Design review of the part built by this model. Coordinates are the model's own, in mm. A direction names the side the tool comes from. Give positions to 0.01 mm unless a question says otherwise; leave off trailing zeros. Order: outer loops, then holes, each group sorted by start corner. A loop starts at its lowest first (then second) coordinate and runs counter-clockwise, first axis right, second up. Notation, with made-up numbers: (-5, 75.25) -> (-1, 75.25) arc R18 ccw to (-1, 86.25) -> close; hole circle Ø9 at (-9.5, -14). An arc over 180 degrees is marked (long way). Use a Markdown table: item, result. Add a question column.
```python
from build123d import *

# Parameters (mm, degrees)
SKETCH1_R           = 4.7625
SKETCH1_R_2         = 1.65
BOSS_EXTRUDE1_DEPTH = 15
SKETCH2_R           = 4.7625
BOSS_EXTRUDE2_DEPTH = 7.5
CUT_EXTRUDE1_REACH  = 66.755
SKETCH3_R           = 2


with BuildPart() as part:
    # Sketch1 → Boss-Extrude1 (new body, symmetric)
    with BuildSketch(Plane.XY):
        with BuildLine():
            Line((-13.253372163, -1.044486042), (-7.531237528, -10.955513958))
            ThreePointArc((-7.531237528, -10.955513958), (-6.784217233, -11.816359568), (-5.770008435, -12.336431676))
            Line((-5.770008435, -12.336431676), (-0.836847118, -13.76941319))
            ThreePointArc((-0.836847118, -13.76941319), (0, -13.888495471), (0.836847118, -13.76941319))
            Line((0.836847118, -13.76941319), (5.770008435, -12.336431676))
            ThreePointArc((5.770008435, -12.336431676), (6.784217233, -11.816359568), (7.531237528, -10.955513958))
            Line((7.531237528, -10.955513958), (13.253372163, -1.044486042))
            ThreePointArc((13.253372163, -1.044486042), (13.625376182, 0.032875315), (13.568667441, 1.171241953))
            Line((13.568667441, 1.171241953), (12.343085176, 6.159975731))
            ThreePointArc((12.343085176, 6.159975731), (12.027789898, 6.944247736), (11.506238058, 7.609437458))
            Line((11.506238058, 7.609437458), (7.798659006, 11.165189723))
            ThreePointArc((7.798659006, 11.165189723), (6.841158949, 11.783484253), (5.722134635, 12))
            Line((5.722134635, 12), (-5.722134635, 12))
            ThreePointArc((-5.722134635, 12), (-6.841158949, 11.783484253), (-7.798659006, 11.165189723))
            Line((-7.798659006, 11.165189723), (-11.506238058, 7.609437458))
            ThreePointArc((-11.506238058, 7.609437458), (-12.027789898, 6.944247736), (-12.343085176, 6.159975731))
            Line((-12.343085176, 6.159975731), (-13.568667441, 1.171241953))
            ThreePointArc((-13.568667441, 1.171241953), (-13.625376182, 0.032875315), (-13.253372163, -1.044486042))
        make_face()
        Circle(SKETCH1_R, mode=Mode.SUBTRACT)
        with Locations((-8.238066653, 4.75625)):
            Circle(SKETCH1_R_2, mode=Mode.SUBTRACT)
        with Locations((8.238066653, 4.75625)):
            Circle(SKETCH1_R_2, mode=Mode.SUBTRACT)
        with Locations((0, -9.5125)):
            Circle(SKETCH1_R_2, mode=Mode.SUBTRACT)
    extrude(amount=BOSS_EXTRUDE1_DEPTH, both=True)

    # Sketch2 → Boss-Extrude2 (add, symmetric)
    with BuildSketch(Plane.XY):
        with BuildLine():
            Line((-12.421472807, 5.666457921), (-9.735682804, 41.826981922))
            ThreePointArc((-9.735682804, 41.826981922), (0, 50.866372944), (9.735682804, 41.826981922))
            Line((9.735682804, 41.826981922), (12.421472807, 5.666457921))
            Line((12.421472807, 5.666457921), (0, 12))
            Line((0, 12), (-12.421472807, 5.666457921))
        make_face()
        with Locations((0, 41.103872944)):
            Circle(SKETCH2_R, mode=Mode.SUBTRACT)
    extrude(amount=BOSS_EXTRUDE2_DEPTH, both=True)

    # Sketch3 → Cut-Extrude1 (cut, up to next)
    with BuildSketch(Plane(origin=(0, 50.866372944, 0), x_dir=(1, 0, 0), z_dir=(0, 1, 0)), mode=Mode.PRIVATE) as cut_extrude1_sk1:
        Circle(SKETCH3_R)
    cut_extrude1_tool1 = extrude(cut_extrude1_sk1.sketch, amount=-CUT_EXTRUDE1_REACH, mode=Mode.PRIVATE) & part.part
    add(cut_extrude1_tool1.solids().sort_by_distance((0, 50.866373, 0))[0], mode=Mode.SUBTRACT)


solid = part.part
```
1) The part is to be moulded in two halves that separate along X. For faces 6 (the cylindrical face through (6.772, -11.826, 0.21)), 7 (the cylindrical face through (-0.215, -7.877, -0.21)), 8 (the cylindrical face through (-6.797, -11.806, 0.21)), 9 (the cylindrical face through (-3.78, -2.9, -0.21)), say which applies: +X half, -X half, draft (parallel to the pull), parting line (faces both ways), or undercut.
2) Insertion check: pin 1 (12 mm diameter, centred on x = 11, z = -1, fed in from -Y); pin 2 (2 mm diameter, centred on x = 0, y = -9.51, fed in from -Z); pin 3 (4 mm diameter, centred on y = 37, z = 7.5, fed in from -X); pin 4 (7.5 mm diameter, centred on x = -2, y = 18.5, fed in from +Z). Each pin has a flat end and moves straight along its axis. Give the tip position at first contact, or say it passes through.
3) Add section A-A (x = 0). Give the boundary of the cut face in (y, z).
4) For L1, parallel to Y at x = 1, z = -3; L2, parallel to Z at x = 0.25, y = 48.5; L3, parallel to Y at x = 0.5, z = -5.5, list the stretches that pass through material, from the lowest coordinate up. Write a range as [from, to].
5) Add section B-B (z = -4). Give the number of separate pieces and of enclosed holes in the cut face, then the cut area to 3 significant figures.
6) Machinability: for faces 1 (the cylindrical face through (-12.022, 6.955, -11.198)), 2 (the cylindrical face through (6.856, 11.777, -11.198)), 3 (the flat face through (-9.63, 9.41, 11.3)), 4 (the cylindrical face through (6.856, 11.777, 11.302)), 5 (the flat face through (0, 12, -11)), which of the approach directions +Z, -Z, +X, -X, +Y, -Y give a long, thin tool a straight path to every point of the face, cutting with its end or side? Answer none if there is none.
7) Add section C-C (y = 0). Give the boundary of the cut face in (x, z).
Worked answers:
| question | item | result |
|---|---|---|
| 1 | face 6 | +X half |
| 1 | face 7 | undercut |
| 1 | face 8 | -X half |
| 1 | face 9 | undercut |
| 2 | pin 1 | y = -12.56 |
| 2 | pin 2 | through |
| 2 | pin 3 | x = -10.24 |
| 2 | pin 4 | z = 7.5 |
| 3 | outline | (-13.89, -15) -> (-11.16, -15) -> (-11.16, 15) -> (-13.89, 15) -> close; (-7.86, -15) -> (-4.76, -15) -> (-4.76, 15) -> (-7.86, 15) -> close; (4.76, -15) -> (12, -15) -> (12, -7.5) -> (36.34, -7.5) -> (36.34, 7.5) -> (12, 7.5) -> (12, 15) -> (4.76, 15) -> close; (45.87, -7.5) -> (50.87, -7.5) -> (50.87, -2) -> (45.87, -2) -> close; (45.87, 2) -> (50.87, 2) -> (50.87, 7.5) -> (45.87, 7.5) -> close |
| 4 | L1 | [-13.72, -10.82], [-8.2, -4.66], [4.66, 36.45], [45.76, 50.82] |
| 4 | L2 | [-7.5, -1.98], [1.98, 7.5] |
| 4 | L3 | [-13.85, -11.08], [-7.94, -4.74], [4.74, 36.37], [45.84, 50.85] |
| 5 | separate pieces | 1 |
| 5 | enclosed holes | 5 |
| 5 | area | 1,180 mm^2 |
| 6 | face 1 | -Z, -X, +Y |
| 6 | face 2 | -Z, +X, +Y |
| 6 | face 3 | +Z, -X, +Y |
| 6 | face 4 | +Z, +X, +Y |
| 6 | face 5 | -Z, +X, -X, +Y |
| 7 | outline | (-13.62, -15) -> (-4.76, -15) -> (-4.76, 15) -> (-13.62, 15) -> close; (4.76, -15) -> (13.62, -15) -> (13.62, 15) -> (4.76, 15) -> close |
